Verification items for the finished model (mm, model axes). A direction names the side the tool comes from. Coordinates: 2 decimals unless noted, no trailing zeros. Write each loop counter-clockwise with the first axis right and the second up, starting at its lowest first coordinate (ties: lowest second). Pieces come first, ordered by that corner, then holes. Notation, with made-up numbers: M -17.75,42.25 L 24.25,42.25 A20 cw 24.25,81.25 Z; hole C 55,5 d5. An arc over 180 degrees is marked long. Answer in a Markdown table with one row per item.
from build123d import *

# Parameters (mm, degrees)
BOSS_EXTRUDE1_DEPTH = 13.5
SKETCH2_W           = 45
SKETCH2_H           = 45
CUT_EXTRUDE1_DEPTH  = 11.72
SKETCH3_R           = 13.5
CUT_EXTRUDE2_DEPTH  = 84.329160712
CHAMFER1_SIZE       = 3
SKETCH7_W           = 113.25
SKETCH7_H           = 1.5
CUT_EXTRUDE4_DEPTH  = 84.598089841
SKETCH5_R           = 1.75
CUT_EXTRUDE7_DEPTH  = 84.013934059
BOSS_EXTRUDE2_START = 5
BOSS_EXTRUDE2_DEPTH = 20
CUT_EXTRUDE8_START  = -30
SKETCH11_W          = 111.517949192
SKETCH11_H          = 10.6
CUT_EXTRUDE8_DEPTH  = 30
SKETCH12_R          = 2
CUT_EXTRUDE9_DEPTH  = 83.19679585
SKETCH13_R          = 3.7
CUT_EXTRUDE10_DEPTH = 9.25
SKETCH14_R          = 83
CUT_EXTRUDE11_DEPTH = 9.25
FILLET1_R           = 5
SKETCH15_W          = 65
SKETCH15_H          = 8
CUT_EXTRUDE12_DEPTH = 9.25
FILLET2_R           = 2
SKETCH16_W          = 23.258974596
SKETCH16_H          = 14
BOSS_EXTRUDE3_DEPTH = 4.7
FILLET3_R           = 5
BOSS_EXTRUDE4_START = 1.5
SKETCH17_R          = 1.75
SKETCH17_R_2        = 13.5
BOSS_EXTRUDE4_DEPTH = 1.5
SKETCH18_W          = 153.260867966
SKETCH18_H          = 50.841882228
CUT_EXTRUDE13_DEPTH = 5


with BuildPart() as part:
    # Sketch1 → Boss-Extrude1 (new body)
    with BuildSketch(Plane(origin=(0, 0, 0), x_dir=(1, 0, 0), z_dir=(0, 1, 0))):
        Polygon((-56.625, 0), (56.625, 0), (21.983983849, 60), (-21.983983849, 60), align=None)
    extrude(amount=BOSS_EXTRUDE1_DEPTH)

    # Sketch2 → Cut-Extrude1 (cut)
    with BuildSketch(Plane.XZ):
        with Locations((0, -31.45)):
            Rectangle(SKETCH2_W, SKETCH2_H)
    extrude(amount=-CUT_EXTRUDE1_DEPTH, mode=Mode.SUBTRACT)

    # Sketch3 → Cut-Extrude2 (cut, through all)
    with BuildSketch(Plane.XZ.offset(-11.72)):
        with Locations(Location((0, -31.45, 0), (0, 0, 270))):
            Circle(SKETCH3_R)
    extrude(amount=-CUT_EXTRUDE2_DEPTH, mode=Mode.SUBTRACT)

    # Chamfer1
    chamfer1_edges = [part.edges().sort_by_distance(p)[0] for p in [
        (-22.5, 5.86, -8.95),
        (-22.5, 5.86, -53.95),
        (22.5, 5.86, -53.95),
        (22.5, 5.86, -8.95),
    ]]
    chamfer(chamfer1_edges, length=CHAMFER1_SIZE)

    # Sketch7 → Cut-Extrude4 (cut, through all)
    with BuildSketch(Plane(origin=(0, 13.5, 0), x_dir=(1, 0, 0), z_dir=(0, 1, 0))):
        with Locations((0, 0.75)):
            Rectangle(SKETCH7_W, SKETCH7_H)
    extrude(amount=-CUT_EXTRUDE4_DEPTH, mode=Mode.SUBTRACT)

    # Sketch5 → Cut-Extrude7 (cut, through all)
    with BuildSketch(Plane(origin=(0, 13.5, 0), x_dir=(1, 0, 0), z_dir=(0, 1, 0))):
        with Locations(Location((15.5, 46.95, 0), (0, 0, 270))):
            Circle(SKETCH5_R)
        with Locations(Location((15.5, 15.95, 0), (0, 0, 270))):
            Circle(SKETCH5_R)
        with Locations(Location((-15.5, 15.95, 0), (0, 0, 270))):
            Circle(SKETCH5_R)
        with Locations(Location((-15.5, 46.95, 0), (0, 0, 270))):
            Circle(SKETCH5_R)
    extrude(amount=-CUT_EXTRUDE7_DEPTH, mode=Mode.SUBTRACT)

    # Sketch10 → Boss-Extrude2 (add)
    with BuildSketch(Plane.XZ.offset(BOSS_EXTRUDE2_START)):
        Polygon((51.457715091, -8.95), (-51.457715091, -8.95), (-55.758974596, -1.5), (-55.758974596, 6.5), (-32.5, 6.5), (-32.5, 28.5), (32.5, 28.5), (32.5, 6.5), (55.758974596, 6.5), (55.758974596, -1.5), align=None)
    extrude(amount=-BOSS_EXTRUDE2_DEPTH)

    # Sketch11 → Cut-Extrude8 (cut)
    with BuildSketch(Plane.XY.offset(28.5).offset(CUT_EXTRUDE8_START)):
        with Locations((0, 5)):
            Rectangle(SKETCH11_W, SKETCH11_H)
    extrude(amount=CUT_EXTRUDE8_DEPTH, mode=Mode.SUBTRACT)

    # Sketch12 → Cut-Extrude9 (cut, through all)
    with BuildSketch(Plane.XY.offset(-1.5)):
        with Locations((-40, 5.15)):
            Circle(SKETCH12_R)
        with Locations((40, 5.15)):
            Circle(SKETCH12_R)
    extrude(amount=-CUT_EXTRUDE9_DEPTH, mode=Mode.SUBTRACT)

    # Sketch13 → Cut-Extrude10 (cut)
    with BuildSketch(Plane.XY.offset(-1.5)):
        with Locations((-40, 5.15)):
            Circle(SKETCH13_R)
        with Locations((40, 5.15)):
            Circle(SKETCH13_R)
    extrude(amount=-CUT_EXTRUDE10_DEPTH, mode=Mode.SUBTRACT)

    # Sketch14 → Cut-Extrude11 (cut)
    with BuildSketch(Plane(origin=(0, 15, 0), x_dir=(1, 0, 0), z_dir=(0, 1, 0))):
        with Locations((0, -98.5)):
            Circle(SKETCH14_R)
    extrude(amount=-CUT_EXTRUDE11_DEPTH, mode=Mode.SUBTRACT)

    # Fillet1
    fillet1_edges = [part.edges().sort_by_distance(p)[0] for p in [
        (-32.5, 12.65, 6.5),
        (32.5, 12.65, 6.5),
        (32.5, -2.65, 6.5),
        (-32.5, -2.65, 6.5),
    ]]
    fillet(fillet1_edges, radius=FILLET1_R)

    # Sketch15 → Cut-Extrude12 (cut)
    with BuildSketch(Plane.XZ.offset(5)):
        with Locations((0, 24.5)):
            Rectangle(SKETCH15_W, SKETCH15_H)
    extrude(amount=-CUT_EXTRUDE12_DEPTH, mode=Mode.SUBTRACT)

    # Fillet2
    fillet2_edges = [part.edges().sort_by_distance(p)[0] for p in [
        (-55.758974596, 12.65, 6.5),
        (55.758974596, 12.65, 6.5),
        (-32.5, 12.65, 22.127557326),
        (32.5, 12.65, 22.127557326),
    ]]
    fillet(fillet2_edges, radius=FILLET2_R)

    # Sketch16 → Boss-Extrude3 (add)
    with BuildSketch(Plane.XZ.offset(5)):
        with Locations((-44.129487298, 13.5)):
            Rectangle(SKETCH16_W, SKETCH16_H)
        with Locations((44.129487298, 13.5)):
            Rectangle(SKETCH16_W, SKETCH16_H)
    extrude(amount=-BOSS_EXTRUDE3_DEPTH)

    # Fillet3
    fillet3_edges = [part.edges().sort_by_distance(p)[0] for p in [
        (-55.758974596, -2.65, 20.5),
        (55.758974596, -2.65, 20.5),
    ]]
    fillet(fillet3_edges, radius=FILLET3_R)

    # Sketch17 → Boss-Extrude4 (add)
    with BuildSketch(Plane(origin=(0, 13.5, 0), x_dir=(1, 0, 0), z_dir=(0, 1, 0)).offset(BOSS_EXTRUDE4_START)):
        Polygon((-51.457715091, 8.95), (51.457715091, 8.95), (21.983983849, 60), (-21.983983849, 60), align=None)
        with Locations(Location((-15.5, 15.95, 0), (0, 0, 270))):
            Circle(SKETCH17_R, mode=Mode.SUBTRACT)
        with Locations(Location((-15.5, 46.95, 0), (0, 0, 270))):
            Circle(SKETCH17_R, mode=Mode.SUBTRACT)
        with Locations(Location((15.5, 46.95, 0), (0, 0, 270))):
            Circle(SKETCH17_R, mode=Mode.SUBTRACT)
        with Locations(Location((15.5, 15.95, 0), (0, 0, 270))):
            Circle(SKETCH17_R, mode=Mode.SUBTRACT)
        with Locations(Location((0, 31.45, 0), (0, 0, 90))):
            Circle(SKETCH17_R_2, mode=Mode.SUBTRACT)
    extrude(amount=-BOSS_EXTRUDE4_DEPTH)

    # Sketch18 → Cut-Extrude13 (cut)
    with BuildSketch(Plane.XZ.offset(5)):
        with Locations((-0.752597738, 9.037202)):
            Rectangle(SKETCH18_W, SKETCH18_H)
    extrude(amount=-CUT_EXTRUDE13_DEPTH, mode=Mode.SUBTRACT)


solid = part.part
1) Thickness scan on L1, parallel to Y at x = -40, z = -5; L2, parallel to X at y = 1.75, z = -3; L3, parallel to X at y = 5.15, z = -25.5. Record the ranges inside material, lowest first. Write a range as [from, to].
Response values:
| item | result |
|---|---|
| L1 | y = [0, 1.45], [8.85, 15] |
| L2 | x = [-54.89, -41.46], [-38.54, 38.54], [41.46, 54.89] |
| L3 | x = [-38, -22.5], [22.5, 38] |
2) Sectioned sample at C-C (z = -29.5). Record the cut outline in (x, y).
Response values:
| item | result |
|---|---|
| outline | M -39.59,0 L -22.5,0 L -22.5,11.72 L -13.36,11.72 L -13.36,15 L -39.59,15 L -39.59,7.11 A2 cw -39.59,3.19 Z; M 13.36,11.72 L 22.5,11.72 L 22.5,0 L 39.59,0 L 39.59,3.19 A2 cw 39.59,7.11 L 39.59,15 L 13.36,15 Z |
3) Release check for a two-part mould opening along Z. For faces 1 (the face through (-32.5, 13, 15)), 2 (the face through (-20.98, 5.78, -10.43)), 3 (the face through (-31.61, 12.683, 20.824)), 4 (the face through (-10, 11.72, -21)) record: +Z half, -Z half, draft (parallel to the pull), parting line (faces both ways), or undercut.
Response values:
| item | result |
|---|---|
| face 1 | draft |
| face 2 | undercut |
| face 3 | +Z half |
| face 4 | undercut |
4) Sectioned sample at D-D (x = 40). Record the cut outline in (y, z), then the cut area to 3 significant figures.
Response values:
| item | result |
|---|---|
| outline | M 0,-28.8 L 3.15,-28.8 L 3.15,-10.75 L 1.45,-10.75 L 1.45,-1.5 L 0,-1.5 Z; M 7.15,-28.8 L 15,-28.8 L 15,6.5 L 10.3,6.5 L 10.3,-1.5 L 8.85,-1.5 L 8.85,-10.75 L 7.15,-10.75 Z |
| area | 306 mm² |
5) Depth check by flat-ended pin: pin 1 (3.5 mm diameter, centred on y = 3.5, z = -25, fed in from +X); pin 2 (1.4 mm diameter, centred on x = -45, y = 12, fed in from +Z); pin 3 (22.5 mm diameter, centred on x = 7, z = -38, fed in from -Y). Enter the tip coordinate at first touch or a pass-through.
Response values:
| item | result |
|---|---|
| pin 1 | stops at x = 43.2 |
| pin 2 | stops at z = 6.5 |
| pin 3 | stops at y = 11.72 |
6) Tool access check on faces 5 (the face through (-46, 13, 6.5)), 6 (the face through (-22.5, 6, -32)), 7 (the face through (42, 4, -10.75)). Record the directions out of +Z, -Z, +X, -X, +Y, -Y that give a thin tool (end or side, any length) a straight path to the whole face; none if there is none.
Response values:
| item | result |
|---|---|
| face 5 | +Z, -X, +Y, -Y |
| face 6 | -Y |
| face 7 | +Z |
7) Sectioned sample at B-B (y = 5.15). Record the cut outline in (x, z).
Response values:
| item | result |
|---|---|
| outline | M -55.76,-1.5 L -42,-25.33 L -42,-10.75 L -43.7,-10.75 L -43.7,-1.5 Z; M -38,-32.26 L -21.98,-60 L 21.98,-60 L 38,-32.26 L 38,-10.75 L 36.3,-10.75 L 36.3,-1.5 L -36.3,-1.5 L -36.3,-10.75 L -38,-10.75 Z; M 42,-25.33 L 55.76,-1.5 L 43.7,-1.5 L 43.7,-10.75 L 42,-10.75 Z; hole M -22.5,-50.95 L -19.5,-53.95 L 19.5,-53.95 L 22.5,-50.95 L 22.5,-11.95 L 19.5,-8.95 L -19.5,-8.95 L -22.5,-11.95 Z |
8) Sectioned sample at A-A (z = -15.95). Record the cut outline in (x, y).
Response values:
| item | result |
|---|---|
| outline | M -47.42,0 L -22.5,0 L -22.5,11.72 L -17.25,11.72 L -17.25,15 L -47.42,15 Z; M -13.75,11.72 L 13.75,11.72 L 13.75,15 L -13.75,15 Z; M 17.25,11.72 L 22.5,11.72 L 22.5,0 L 47.42,0 L 47.42,15 L 17.25,15 Z; hole C -40,5.15 d4; hole C 40,5.15 d4 |
